Geometry: final body of the model. Coordinates: model frame, mm. Face numbers are marked on the shaded views. A direction names the side the tool comes from. Give positions to 0.01 mm unless a question says otherwise; leave off trailing zeros. Loops run counter-clockwise (first coordinate to the right, second up) from the corner with the lowest first, then second, coordinate; pieces in that order, holes last. Notation, with made-up numbers: (-8.75, 62) -> (20.25, 62) arc R17 ccw to (20.25, 95) -> close; hole circle Ø10 at (-7, 61.5). An arc over 180 degrees is marked (long way). Answer in a Markdown table with one row per item. Add a question column.
1) Section query B-B (x = 0.5). Return the cut outline in (y, z), plus the area to 3 significant figures.
2) First-contact query: P1, Ø1.6, axis at y = 9, z = 33.5, coming from the +X side; P2, Ø1, axis at y = 10.5, z = 32.5, coming from the -X side; P3, Ø6, axis at x = -19, z = -15, coming from the +Y side. Flat tips, straight axial feed; report the tip coordinate or a pass-through.
3) Section query D-D (x = -16.5). Return the cut outline in (y, z), plus the area to 3 significant figures.
4) Line query: line 1 (X direction, y = 5.75, z = 7); line 2 (Z direction, x = 12.5, y = 4); line 3 (Y direction, x = 27, z = 5.5). Output: solid intervals per line, ascending. Write a range as from..to.
5) Access query for the marked faces 1 and 2. Directions: +Z, -Z, +X, -X, +Y, -Y. A direction counts if a zero-diameter tool reaches every point of the face in a straight line with its end or side. Return the directions, or none.
6) Section query A-A (y = 10). Return the cut outline in (x, z), plus the area to 3 significant figures.
7) Draft query along X for the marked faces 3, 4 and 5. Return one class per face: +X half, -X half, draft (parallel to the pull), parting line (faces both ways), or undercut.
8) Section query C-C (z = -10). Return the cut outline in (x, y).
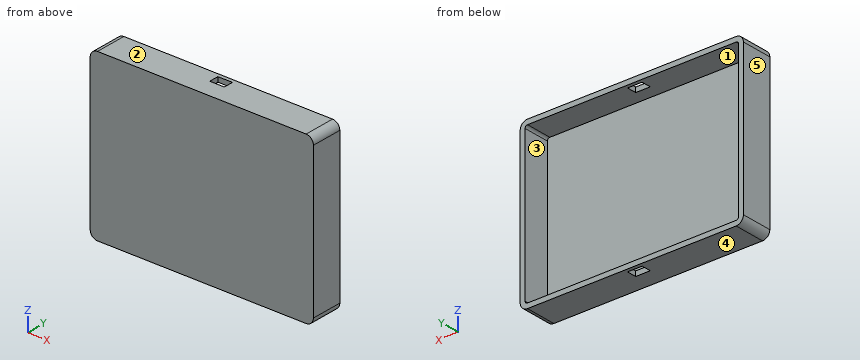
```python
from build123d import *

# Parameters (mm, degrees)
SKETCH1_W               = 92
SKETCH1_H               = 68
BOSS_EXTRUDE1_DEPTH     = 13
FILLET1_R               = 3
SHELL1_T                = -2
SKETCH2_W               = 6
SKETCH2_H               = 4
CUT_EXTRUDE1_DEPTH      = 1
CUT_EXTRUDE1_DEPTH_BACK = 69


with BuildPart() as part:
    # Sketch1 → Boss-Extrude1 (new body)
    with BuildSketch(Plane(origin=(0, 0, 0), x_dir=(1, 0, 0), z_dir=(0, 1, 0))):
        Rectangle(SKETCH1_W, SKETCH1_H)
    extrude(amount=BOSS_EXTRUDE1_DEPTH)

    # Fillet1
    fillet1_edges = [part.edges().sort_by_distance(p)[0] for p in [
        (46, 6.5, 34),
        (-46, 6.5, 34),
        (-46, 6.5, -34),
        (46, 6.5, -34),
    ]]
    fillet(fillet1_edges, radius=FILLET1_R)

    # Shell1
    shell1_openings = [part.faces().sort_by_distance(p)[0] for p in [
        (0, 13, 0),
    ]]
    offset(amount=SHELL1_T, openings=shell1_openings, kind=Kind.INTERSECTION)

    # Sketch2 → Cut-Extrude1 (cut, two sides)
    with BuildSketch(Plane.XY.offset(34)) as cut_extrude1_sk:
        with Locations((0, 9.5)):
            Rectangle(SKETCH2_W, SKETCH2_H)
    extrude(amount=CUT_EXTRUDE1_DEPTH, mode=Mode.SUBTRACT)
    extrude(cut_extrude1_sk.sketch, amount=-CUT_EXTRUDE1_DEPTH_BACK, mode=Mode.SUBTRACT)


solid = part.part
```
Evaluation:
| question | item | result |
|---|---|---|
| 1 | outline | (0, -34) -> (7.5, -34) -> (7.5, -32) -> (2, -32) -> (2, 32) -> (7.5, 32) -> (7.5, 34) -> (0, 34) -> close; (11.5, -34) -> (13, -34) -> (13, -32) -> (11.5, -32) -> close; (11.5, 32) -> (13, 32) -> (13, 34) -> (11.5, 34) -> close |
| 1 | area | 164 mm² |
| 2 | P1 | x = 45.47 |
| 2 | P2 | x = -45.83 |
| 2 | P3 | y = 2 |
| 3 | outline | (0, -34) -> (13, -34) -> (13, -32) -> (2, -32) -> (2, 32) -> (13, 32) -> (13, 34) -> (0, 34) -> close |
| 3 | area | 180 mm² |
| 4 | line 1 | -46..-44, 44..46 |
| 4 | line 2 | -34..-32, 32..34 |
| 4 | line 3 | 0..2 |
| 5 | face 1 | +Y |
| 5 | face 2 | +Z, +X, -X, +Y, -Y |
| 6 | outline | (-46, -31) arc R3 ccw to (-43, -34) -> (-3, -34) -> (-3, -32) -> (-43, -32) arc R1 cw to (-44, -31) -> (-44, 31) arc R1 cw to (-43, 32) -> (-3, 32) -> (-3, 34) -> (-43, 34) arc R3 ccw to (-46, 31) -> close; (3, -34) -> (43, -34) arc R3 ccw to (46, -31) -> (46, 31) arc R3 ccw to (43, 34) -> (3, 34) -> (3, 32) -> (43, 32) arc R1 cw to (44, 31) -> (44, -31) arc R1 cw to (43, -32) -> (3, -32) -> close |
| 6 | area | 593 mm² |
| 7 | face 3 | undercut |
| 7 | face 4 | draft |
| 7 | face 5 | -X half |
| 8 | outline | (-46, 0) -> (46, 0) -> (46, 13) -> (44, 13) -> (44, 2) -> (-44, 2) -> (-44, 13) -> (-46, 13) -> close |
